Work out the finished part from the listing and answer in its coordinate system (mm). A direction names the side the tool comes from. Round coordinates to 2 decimals unless told otherwise and drop trailing zeros. Order: outer loops, then holes, each group sorted by start corner. A loop starts at its lowest first (then second) coordinate and runs counter-clockwise, first axis right, second up. Notation, with made-up numbers: (-19, -20.5) - (35, -20.5) arc R17 cw to (35, -15.5) - close; hole circle Ø5 at (24.5, -18). An arc over 180 degrees is marked (long way). Answer in a Markdown table with one row per item.
from build123d import *

# Parameters (mm, degrees)
F0_R     = 10.75
F1_DEPTH = 2.5
F2_R     = 4.05
F3_DEPTH = 5.5
F4_SIZE  = 0.5
F5_R     = 4.55
F6_DEPTH = 2
F7_DEPTH = 0.5


# Not quite as in the source:
# - a feature names something its author has since deleted; it is built from what else it names


with BuildPart() as f1:
    # F0 (on Top) → F1 (new body)
    with BuildSketch(Plane.XY):
        Circle(F0_R)
        with BuildLine():
            ThreePointArc((0, -10), (-7.0710678119, 7.0710678119), (10, 0))
            ThreePointArc((10, 0), (7.0710678119, -7.0710678119), (0, -10))
        make_face(mode=Mode.SUBTRACT)
        with BuildLine():
            ThreePointArc((0, -10), (7.0710678119, -7.0710678119), (10, 0))
            ThreePointArc((10, 0), (-7.0710678119, 7.0710678119), (0, -10))
        make_face()
        Polygon((3.1044567973, -4.3237269842), (0, -10), (-3.1044567973, -4.3237269842), (-9.4622431459, -3.1252779442), (-5.0231166146, 1.581300749), (-5.847987874, 7.9982560054), (0, 5.2308085927), (5.847987874, 7.9982560054), (5.0231166146, 1.581300749), (9.4622431459, -3.1252779442), align=None, mode=Mode.SUBTRACT)
        Polygon((-3.1044567973, -4.3237269842), (0, -10), (3.1044567973, -4.3237269842), (9.4622431459, -3.1252779442), (5.0231166146, 1.581300749), (5.847987874, 7.9982560054), (0, 5.2308085927), (-5.847987874, 7.9982560054), (-5.0231166146, 1.581300749), (-9.4622431459, -3.1252779442), align=None)
    extrude(amount=F1_DEPTH)

    # F2 (on face) → F3 (join)
    with BuildSketch(Plane.XY.offset(2.5)):
        Circle(F2_R)
    extrude(amount=F3_DEPTH)

    # F4
    f4_edges = [f1.edges().sort_by_distance(p)[0] for p in [
        (-4.05, 0, 8),
    ]]
    chamfer(f4_edges, length=F4_SIZE)

    # F5 (on face) → F6 (join)
    with BuildSketch(Plane.XY.offset(2.5)):
        Circle(F5_R)
    extrude(amount=F6_DEPTH)

    # F0 (on Top) → F7 (cut)
    with BuildSketch(Plane.XY):
        Polygon((-3.1044567973, -4.3237269842), (0, -10), (3.1044567973, -4.3237269842), (9.4622431459, -3.1252779442), (5.0231166146, 1.581300749), (5.847987874, 7.9982560054), (0, 5.2308085927), (-5.847987874, 7.9982560054), (-5.0231166146, 1.581300749), (-9.4622431459, -3.1252779442), align=None)
    extrude(amount=F7_DEPTH, mode=Mode.SUBTRACT)


solid = f1.part
1) The mould has two halves that part along Y. Classify faces 4 (the face through (5.43, 4.74, 0.25)), 5 (the face through (-0.99, -4.44, 3.49)), 6 (the face through (5, -5, 0)): released by +Y, released by -Y, zero draft, split by the parting line, or undercut.
Filled in:
| item | result |
|---|---|
| face 4 | undercut |
| face 5 | split by the parting line |
| face 6 | zero draft |
2) Which of the six approach directions +Z, -Z, +X, -X, +Y, -Y give full straight-line access (tool end or side, diameter ignored) to faces 1 (the face through (-1.4, 10.66, 1.23)), 2 (the face through (-0.878, -3.954, 5.979)), 3 (the face through (-1.574, -7.122, 0.246))?
Filled in:
| item | result |
|---|---|
| face 1 | +Z, -Z |
| face 2 | +Z |
| face 3 | -Z |
3) Each of these flat-tipped pins is pushed along its axis until it touches: pin 1 (3 mm diameter, centred on y = -7, z = 3, fed in from -X); pin 2 (1.5 mm diameter, centred on y = 3, z = 1.5, fed in from -X); pin 3 (3 mm diameter, centred on x = -8.5, z = 5, fed in from -Y); pin 4 (3 mm diameter, centred on x = 0, z = 6.5, fed in from -Y). Where does it stop, or does it pass through?
Filled in:
| item | result |
|---|---|
| pin 1 | stops at x = -9.18 |
| pin 2 | stops at x = -10.51 |
| pin 3 | passes through |
| pin 4 | stops at y = -4.05 |
4) Find section C-C, the plane y = 0. Give the vertices of the cut face in (x, z).
Filled in:
| item | result |
|---|---|
| outline | (-10.75, 0) - (-6.51, 0) - (-6.51, 0.5) - (6.51, 0.5) - (6.51, 0) - (10.75, 0) - (10.75, 2.5) - (4.55, 2.5) - (4.55, 4.5) - (4.05, 4.5) - (4.05, 7.5) - (3.55, 8) - (-3.55, 8) - (-4.05, 7.5) - (-4.05, 4.5) - (-4.55, 4.5) - (-4.55, 2.5) - (-10.75, 2.5) - close |
5) Find the intervals of material crossed by probe 1 along Z at (x, y) = (-0.5, -9.25); probe 2 along X at (y, z) = (-9.5, 2); probe 3 along Z at (x, y) = (0, -6.25), in increasing order. Write a range as from..to.
Filled in:
| item | result |
|---|---|
| probe 1 | z = 0..2.5 |
| probe 2 | x = -5.03..5.03 |
| probe 3 | z = 0.5..2.5 |
6) Find section B-B, the plane z = 4. Give the vertices of the cut face in (x, y).
Filled in:
| item | result |
|---|---|
| outline | circle Ø9.1 at (0, 0) |
7) Find section A-A, the plane x = 9. Give the vertices of the cut face in (y, z).
Filled in:
| item | result |
|---|---|
| outline | (-5.88, 0) - (-3.21, 0) - (-3.21, 0.5) - (-2.64, 0.5) - (-2.64, 0) - (5.88, 0) - (5.88, 2.5) - (-5.88, 2.5) - close |
8) Find section D-D, the plane x = -7.5. Give the vertices of the cut face in (y, z).
Filled in:
| item | result |
|---|---|
| outline | (-7.7, 0) - (-3.5, 0) - (-3.5, 0.5) - (-1.04, 0.5) - (-1.04, 0) - (7.7, 0) - (7.7, 2.5) - (-7.7, 2.5) - close |
